The model under review builds one solid part; all positions refer to its coordinate system, in mm. A direction names the side the tool comes from. Round coordinates to 2 decimals unless told otherwise and drop trailing zeros. Order: outer loops, then holes, each group sorted by start corner. A loop starts at its lowest first (then second) coordinate and runs counter-clockwise, first axis right, second up. Notation, with made-up numbers: (28.25, 86) - (48.25, 86) arc R28 cw to (48.25, 104) - close; hole circle Ø4 at (-14, 69.5). An arc over 180 degrees is marked (long way). One line per question, with ' | ' between items. Start each with the question number.
Item 1: For L1, parallel to Z at x = 2.7, y = 0; L2, parallel to Z at x = 3.65, y = -4; L3, parallel to Z at x = 0.45, y = 3.75, list the stretches that pass through material, from the lowest coordinate up. Write a range as [from, to].
Item 2: Draft analysis for pull direction Y (two halves, no side actions). For faces 4 (the face through (0.25, 5.27, 5.75)), 5 (the face through (2.028, 4.57, 7.167)), 6 (the face through (4, -4, -7)), state which applies: +Y half, -Y half, draft (parallel to the pull), parting line (faces both ways), or undercut.
Item 3: Insertion check: pin 1 Ø5 at (y, z) = (5.5, 1.5) entering from -X; pin 2 Ø1.5 at (x, z) = (2, -6) entering from -Y. Each pin has a flat end and moves straight along its axis. Give the tip position at first contact, or say it passes through.
Item 4: Add section C-C on x = 3.25. State the section outline as (y, z) points.
Item 5: Tool access review of faces 1 (the face through (0.5, -2, -5)), 2 (the face through (0, -4, -7)), 3 (the face through (3.5, -2, -5)): name each direction out of +Z, -Z, +X, -X, +Y, -Y from which nothing blocks a thin tool from reaching the whole face with its end or side.
Item 6: Add section D-D on y = 6.25. State the section outline as (x, z) points, and give its area (3 significant figures).
Item 7: Add section A-A on z = 0. State the section outline as (x, y) points, and give its area (3 significant figures).
from build123d import *

# Parameters (mm, degrees)
CROQUIS1_W            = 4
CROQUIS1_H            = 4
CROQUIS2_R            = 7.8
CROQUIS2_R_2          = 5.2
CORTAR_EXTRUIR1_DEPTH = 0.5


with BuildPart() as part:
    # Croquis1 → Revolución1 (revolve)
    with BuildSketch(Plane.XY):
        with Locations((2, 6.5)):
            Rectangle(CROQUIS1_W, CROQUIS1_H)
    revolve(axis=Axis((0, 0, 0), (1, 0, 0)))

    # Croquis2 → Cortar-Extruir1 (cut)
    with BuildSketch(Plane(origin=(4, 0, 0), x_dir=(0, 0, -1), z_dir=(1, 0, 0))):
        Circle(CROQUIS2_R)
        Circle(CROQUIS2_R_2, mode=Mode.SUBTRACT)
    cortar_extruir1 = extrude(amount=-CORTAR_EXTRUIR1_DEPTH, mode=Mode.SUBTRACT)

    # Simetría1: Cortar-Extruir1 across plane
    add(cortar_extruir1.mirror(Plane(origin=(2, 0, 0), x_dir=(0, 0, 1), z_dir=(1, 0, 0))), mode=Mode.SUBTRACT)


solid = part.part
Determined:
1) L1: [-8.5, -4.5], [4.5, 8.5] | L2: [-7.5, -6.7], [-3.32, -2.06], [2.06, 3.32], [6.7, 7.5] | L3: [-7.63, -6.84], [-3.6, -2.49], [2.49, 3.6], [6.84, 7.63]
2) face 4: undercut | face 5: parting line | face 6: draft
3) pin 1: x = 0 | pin 2: y = -6.68
4) outline: circle Ø17 at (0, 0); hole circle Ø9 at (0, 0)
5) face 1: -X | face 2: +Z, -Z, -X, +Y, -Y | face 3: +X
6) outline: (0, -5.76) - (4, -5.76) - (4, -4.67) - (3.5, -4.67) - (3.5, 4.67) - (4, 4.67) - (4, 5.76) - (0, 5.76) - (0, 4.67) - (0.5, 4.67) - (0.5, -4.67) - (0, -4.67) - close | area: 36.8 mm2
7) outline: (0, -8.5) - (4, -8.5) - (4, -7.8) - (3.5, -7.8) - (3.5, -5.2) - (4, -5.2) - (4, -4.5) - (0, -4.5) - (0, -5.2) - (0.5, -5.2) - (0.5, -7.8) - (0, -7.8) - close; (0, 4.5) - (4, 4.5) - (4, 5.2) - (3.5, 5.2) - (3.5, 7.8) - (4, 7.8) - (4, 8.5) - (0, 8.5) - (0, 7.8) - (0.5, 7.8) - (0.5, 5.2) - (0, 5.2) - close | area: 26.8 mm2
